Geometry check sheet. Reference: drawing and pictorial views, mm from the part's lowest x, y, z. A direction names the side the tool comes from. Give positions to 0.01 mm unless a question says otherwise; leave off trailing zeros. Write each loop counter-clockwise with the first axis right and the second up, starting at its lowest first coordinate (ties: lowest second). Pieces come first, ordered by that corner, then holes. Notation, with made-up numbers: (86, -38) -> (132, -38) arc R21 cw to (132, -20) -> close; hole circle Ø6 at (-34.75, -14). An arc over 180 degrees is marked (long way). Return JSON: item names as keys, results as strings.
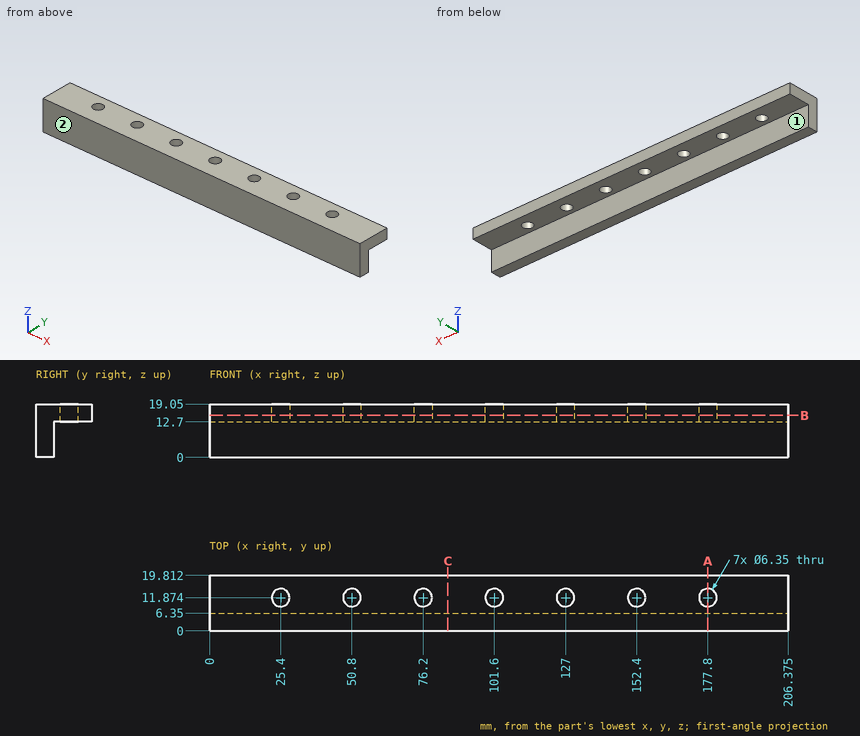
(1) Set-up check for the marked faces 1 and 2: record each of +Z, -Z, +X, -X, +Y, -Y from which the full face is reachable in a straight line by a thin tool's end or side.
Reply:
{"face 1": "-Z, +X, -X, +Y", "face 2": "+Z, -Z, +X, -X, -Y"}
(2) Depth check by flat-ended pin: pin 1 Ø4 at (x, y) = (89, 12) entering from -Z. Enter the tip coordinate at first touch or a pass-through.
Reply:
{"pin 1": "z = 12.7"}
(3) Cross-section at A-A on x = 177.8. Enter the section's corners in (y, z).
Reply:
{"outline": "(0, 0) -> (6.35, 0) -> (6.35, 12.7) -> (8.7, 12.7) -> (8.7, 19.05) -> (0, 19.05) -> close; (15.05, 12.7) -> (19.81, 12.7) -> (19.81, 19.05) -> (15.05, 19.05) -> close"}
(4) Cross-section at C-C on x = 85. Enter the section's corners in (y, z).
Reply:
{"outline": "(0, 0) -> (6.35, 0) -> (6.35, 12.7) -> (19.81, 12.7) -> (19.81, 19.05) -> (0, 19.05) -> close"}
(5) Thickness scan on L1, parallel to Y at x = 127, z = 14.5; L2, parallel to Y at x = 67, z = 7.25; L3, parallel to Z at x = 14, y = 15. Record the ranges inside material, lowest first.
Reply:
{"L1": "0 to 8.7, 15.05 to 19.81", "L2": "0 to 6.35", "L3": "12.7 to 19.05"}
(6) Cross-section at B-B on z = 15. State how many separate pieces and enclosed holes the cut face has, then the cut area to 3 significant figures.
Reply:
{"separate pieces": "1", "enclosed holes": "7", "area": "3,870 mm^2"}
